Build history of the part. All positions in model axes, mm. A direction names the side the tool comes from. Round coordinates to 2 decimals unless told otherwise and drop trailing zeros. Loops run counter-clockwise (first coordinate to the right, second up) from the corner with the lowest first, then second, coordinate; pieces in that order, holes last. Notation, with made-up numbers: (43.25, -27) - (83.25, -27) arc R22 cw to (83.25, 10) - close; hole circle Ø6 at (18, 27). An arc over 180 degrees is marked (long way). Use a Markdown table: item, result.
from build123d import *

# Parameters (mm, degrees)
SKETCH1_W                                        = 174.796166906
SKETCH1_H                                        = 108.92723011
BOSS_EXTRUDE1_DEPTH                              = 43.18
SKETCH2_R                                        = 7.697413188
SKETCH2_R_2                                      = 9.430807524
CUT_EXTRUDE1_DEPTH                               = 12.7
CUT_EXTRUDE2_DEPTH                               = 10
CSK_FOR_M10_FLAT_HEAD_MACHINE_SCREW1_D           = 11
CSK_FOR_M10_FLAT_HEAD_MACHINE_SCREW1_DEPTH       = 16.695266595
CSK_FOR_M10_FLAT_HEAD_MACHINE_SCREW1_CSINK_D     = 20
CSK_FOR_M10_FLAT_HEAD_MACHINE_SCREW1_CSINK_ANGLE = 90
CSK_FOR_M10_FLAT_HEAD_MACHINE_SCREW1_TIP         = 3.304733405
CHAMFER1_SIZE                                    = 3


with BuildPart() as part:
    # Sketch1 → Boss-Extrude1 (new body)
    with BuildSketch(Plane(origin=(0, 0, 0), x_dir=(1, 0, 0), z_dir=(0, 1, 0))):
        Rectangle(SKETCH1_W, SKETCH1_H)
    extrude(amount=BOSS_EXTRUDE1_DEPTH)

    # Sketch2 → Cut-Extrude1 (cut)
    with BuildSketch(Plane(origin=(0, 43.18, 0), x_dir=(1, 0, 0), z_dir=(0, 1, 0))):
        with Locations(Location((-72.874036632, 36.40863105, 0), (0, 0, 270))):  # turned: the seam where the file's is
            Circle(SKETCH2_R)
        with Locations(Location((70.801263176, -36.157833353, 0), (0, 0, 270))):  # turned: the seam where the file's is
            Circle(SKETCH2_R_2)
        with BuildLine():
            Line((-50.8, 12.7), (50.8, 12.7))
            ThreePointArc((50.8, 12.7), (63.5, 0), (50.8, -12.7))
            Line((50.8, -12.7), (-50.8, -12.7))
            ThreePointArc((-50.8, -12.7), (-63.5, 0), (-50.8, 12.7))
        make_face()
    extrude(amount=-CUT_EXTRUDE1_DEPTH, mode=Mode.SUBTRACT)

    # Sketch3 → Cut-Extrude2 (cut)
    with BuildSketch(Plane(origin=(0, 43.18, 0), x_dir=(1, 0, 0), z_dir=(0, 1, 0))):
        with BuildLine():
            Line((10, 36.036384945), (10, -38.963615055))
            ThreePointArc((10, -38.963615055), (0, -48.963615055), (-10, -38.963615055))
            Line((-10, -38.963615055), (-10, 36.036384945))
            ThreePointArc((-10, 36.036384945), (0, 46.036384945), (10, 36.036384945))
        make_face()
    extrude(amount=-CUT_EXTRUDE2_DEPTH, mode=Mode.SUBTRACT)

    # CSK for M10 Flat Head Machine Screw1
    with Locations(Plane(origin=(0, 43.18, 0), x_dir=(1, 0, 0), z_dir=(0, 1, 0))):
        with Locations((67.398083453, 34.463615055), (-67.398083453, -34.463615055)):
            CounterSinkHole(CSK_FOR_M10_FLAT_HEAD_MACHINE_SCREW1_D / 2, CSK_FOR_M10_FLAT_HEAD_MACHINE_SCREW1_CSINK_D / 2, depth=CSK_FOR_M10_FLAT_HEAD_MACHINE_SCREW1_DEPTH, counter_sink_angle=CSK_FOR_M10_FLAT_HEAD_MACHINE_SCREW1_CSINK_ANGLE)
            with Locations((0, 0, -(CSK_FOR_M10_FLAT_HEAD_MACHINE_SCREW1_DEPTH + CSK_FOR_M10_FLAT_HEAD_MACHINE_SCREW1_TIP / 2))):  # 118° drill point
                Cone(0, CSK_FOR_M10_FLAT_HEAD_MACHINE_SCREW1_D / 2, CSK_FOR_M10_FLAT_HEAD_MACHINE_SCREW1_TIP, mode=Mode.SUBTRACT)

    # Chamfer1
    chamfer1_edges = [part.edges().sort_by_distance(p)[0] for p in [
        (-87.398083453, 43.18, 0),
        (0, 43.18, 54.463615055),
        (87.398083453, 43.18, 0),
        (0, 43.18, -54.463615055),
    ]]
    chamfer(chamfer1_edges, length=CHAMFER1_SIZE)


solid = part.part
Q1. Probe line 1 (Z direction, x = 22, y = 36); line 2 (Z direction, x = -57, y = 40.5); line 3 (Y direction, x = 45, z = 1.5). List the from-to ranges inside material, lowest first.
Results found:
| item | result |
|---|---|
| line 1 | z = -54.46 to -12.7, 12.7 to 54.46 |
| line 2 | z = -54.14 to -11.08, 11.08 to 54.14 |
| line 3 | y = 0 to 30.48 |
Q2. Which spindle directions (+Z, -Z, +X, -X, +Y, -Y) get a long thin tool onto all of the face, cutting with end or side? Do faces 1 (the face through (-87.398, 20, 1)), 2 (the face through (71.45, 32.5, -38.18)). Say none if no direction does.
Results found:
| item | result |
|---|---|
| face 1 | +Z, -Z, -X, +Y, -Y |
| face 2 | +Y |
Q3. Cut at A-A, the plane x = 0. List the corners of the cut face in (y, z).
Results found:
| item | result |
|---|---|
| outline | (0, -54.46) - (40.18, -54.46) - (43.18, -51.46) - (43.18, -46.04) - (33.18, -46.04) - (33.18, -12.7) - (30.48, -12.7) - (30.48, 12.7) - (33.18, 12.7) - (33.18, 48.96) - (43.18, 48.96) - (43.18, 51.46) - (40.18, 54.46) - (0, 54.46) - close |
Q4. Cut at C-C, the plane x = -45.5. List the corners of the cut face in (y, z), plus the area to 3 significant figures.
Results found:
| item | result |
|---|---|
| outline | (0, -54.46) - (40.18, -54.46) - (43.18, -51.46) - (43.18, -12.7) - (30.48, -12.7) - (30.48, 12.7) - (43.18, 12.7) - (43.18, 51.46) - (40.18, 54.46) - (0, 54.46) - close |
| area | 4,370 mm2 |
Q5. Pull direction Z, two halves, no side cores. Call faces 3 (the face through (87.398, 20, 1)), 4 (the face through (-1, 20, -54.464)), 5 (the face through (0, 33.18, -30)), 6 (the face through (61.595, 36.919, 34.113)): pulls with the +Z half, pulls with the -Z half, needs draft (parallel to the pull), parting line crosses it, or undercut.
Results found:
| item | result |
|---|---|
| face 3 | needs draft |
| face 4 | pulls with the -Z half |
| face 5 | undercut |
| face 6 | undercut |
Q6. Drop flat-ended pins along their axis: pin 1 (16 mm diameter, centred on x = 1, z = 32, fed in from +Y); pin 2 (7.5 mm diameter, centred on x = -75.5, z = -39, fed in from +Y). Give the stop position or say it passes through.
Results found:
| item | result |
|---|---|
| pin 1 | stops at y = 33.18 |
| pin 2 | stops at y = 30.48 |
Q7. Cut at B-B, the plane z = 0. List the corners of the cut face in (x, y), plus the area to 3 significant figures.
Results found:
| item | result |
|---|---|
| outline | (-87.4, 0) - (87.4, 0) - (87.4, 40.18) - (84.4, 43.18) - (63.5, 43.18) - (63.5, 30.48) - (-63.5, 30.48) - (-63.5, 43.18) - (-84.4, 43.18) - (-87.4, 40.18) - close |
| area | 5,930 mm2 |
